Build history of the part. All positions in model axes, mm. Face numbers are marked on the shaded views. Coordinates: 2 decimals unless noted, no trailing zeros. Order: outer loops, then holes, each group sorted by start corner. A loop starts at its lowest first (then second) coordinate and runs counter-clockwise, first axis right, second up. Notation, with made-up numbers: (-13.5, 60) - (38.5, 60) arc R15 ccw to (38.5, 76) - close; hole circle Ø9 at (70.5, -0.5). An arc over 180 degrees is marked (long way). Write each question's results on one line, items separated by ' | '.
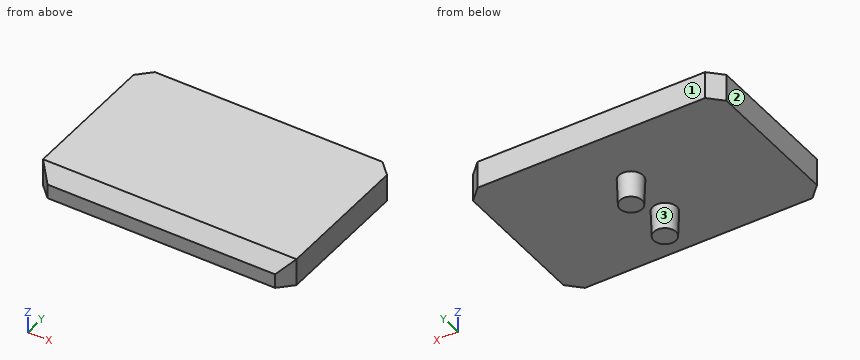
from build123d import *

# Parameters (mm, degrees)
BUTTON_1_DEPTH            = 2.1
SKETCH_1_R                = 0.925
EXTRUDE_1_DEPTH           = 2
EXTRUDE_1_DRAFT           = 2
EXTRUDE_1_PROFILE_2_DEPTH = 2
EXTRUDE_1_PROFILE_2_DRAFT = 2
CHAMFER_1_SIZE            = 1
CHAMFER_2_SIZE            = 1


# Read off the part's stored shape, not the designer's step: 基体零件-button-1
with BuildPart() as part:
    # 基体零件-button-1 outline → 基体零件-button-1 (new body)
    with BuildSketch(Plane.XY):
        Polygon((-62.765330564, -7.006843897), (-62.765330564, -18.706843897), (-61.765330564, -19.706843897), (-44.265330564, -19.706843897), (-43.265330564, -18.706843897), (-43.265330564, -7.006843897), align=None)
    extrude(amount=BUTTON_1_DEPTH)


with BuildPart() as extrude_1_tool:
    # 草图1 → 凸台-拉伸1 (with draft: the straight prism first)
    with BuildSketch(Plane(origin=(0, 0, 0), x_dir=(-1, 0, 0), z_dir=(0, 0, -1))):
        with Locations((53.015330564, -11.706843897)):
            Circle(SKETCH_1_R)
    extrude(amount=EXTRUDE_1_DEPTH)
    # 凸台-拉伸1: the draft: its side faces are tilted about the plane it starts from
    extrude_1_sides = [extrude_1_tool.faces().sort_by_distance(p)[0] for p in [
        (-52.090330564, -11.706843897, -1),
    ]]
    draft(extrude_1_sides, Plane(origin=(0, 0, 0), x_dir=(-1, 0, 0), z_dir=(0, 0, -1)), EXTRUDE_1_DRAFT)


with BuildPart() as part_1:
    add(part.part)

    # 凸台-拉伸1: add extrude_1_tool
    add(extrude_1_tool.part)


with BuildPart() as extrude_1_profile_2_tool:
    # 草图1 → 凸台-拉伸1 profile 2 (with draft: the straight prism first)
    with BuildSketch(Plane(origin=(0, 0, 0), x_dir=(-1, 0, 0), z_dir=(0, 0, -1))):
        with Locations((53.015330564, -15.706843897)):
            Circle(SKETCH_1_R)
    extrude(amount=EXTRUDE_1_PROFILE_2_DEPTH)
    # 凸台-拉伸1 profile 2: the draft: its side faces are tilted about the plane it starts from
    extrude_1_profile_2_sides = [extrude_1_profile_2_tool.faces().sort_by_distance(p)[0] for p in [
        (-52.090330564, -15.706843897, -1),
    ]]
    draft(extrude_1_profile_2_sides, Plane(origin=(0, 0, 0), x_dir=(-1, 0, 0), z_dir=(0, 0, -1)), EXTRUDE_1_PROFILE_2_DRAFT)


with BuildPart() as part_2:
    add(part_1.part)

    # 凸台-拉伸1 profile 2: add extrude_1_profile_2_tool
    add(extrude_1_profile_2_tool.part)

    # 倒角1
    chamfer_1_edges = [part_2.edges().sort_by_distance(p)[0] for p in [
        (-53.015330564, -19.706843897, 2.1),
    ]]
    chamfer(chamfer_1_edges, length=CHAMFER_1_SIZE)

    # 倒角2
    chamfer_2_edges = [part_2.edges().sort_by_distance(p)[0] for p in [
        (-62.765330564, -7.006843897, 1.05),
        (-43.265330564, -7.006843897, 1.05),
    ]]
    chamfer(chamfer_2_edges, length=CHAMFER_2_SIZE)


solid = part_2.part
1. Band-saw the part on D-D on y = -8.5. Give the cut face in (x, z).
Solved:
outline: (-62.77, 0) - (-43.27, 0) - (-43.27, 2.1) - (-62.77, 2.1) - close
2. Band-saw the part on A-A on x = -56.75. Give the cut face in (y, z).
Solved:
outline: (-19.71, 0) - (-7.01, 0) - (-7.01, 2.1) - (-18.71, 2.1) - (-19.71, 1.1) - close
3. Band-saw the part on C-C on z = -0.25. Give the cut face in (x, y).
Solved:
outline: circle Ø1.83 at (-53.02, -15.71); circle Ø1.83 at (-53.02, -11.71)
4. Two-plate mould, pull along Y, no slides. Class the marked faces 1, 2 and 3: +Y half, -Y half, draft (parallel to the pull), parting line (faces both ways), or undercut.
Solved:
face 1: +Y half | face 2: draft | face 3: undercut
5. Probe line 1 (Z direction, x = -54.5, y = -8.5); line 2 (Y direction, x = -61.75, z = 1.35); line 3 (Y direction, x = -58, z = 1.7). List the from-to ranges inside material, lowest first.
Solved:
line 1: z = 0 to 2.1 | line 2: y = -19.46 to -7.01 | line 3: y = -19.11 to -7.01
6. Band-saw the part on B-B on z = 1.6. Give the cut face in (x, y).
Solved:
outline: (-62.77, -18.71) - (-62.27, -19.21) - (-43.77, -19.21) - (-43.27, -18.71) - (-43.27, -8.01) - (-44.27, -7.01) - (-61.77, -7.01) - (-62.77, -8.01) - close
